The listing builds one solid part. Answer for the finished solid, in the listing's coordinates (mm). Face numbers are marked on the shaded views. Coordinates: 2 decimals unless noted, no trailing zeros. Order: outer loops, then holes, each group sorted by start corner. A loop starts at its lowest first (then second) coordinate and runs counter-clockwise, first axis right, second up. Notation, with made-up numbers: (65.5, 28.5) -> (115.5, 28.5) arc R17 ccw to (115.5, 48.5) -> close; hole circle Ø9 at (46, 37.25). An arc over 180 degrees is marked (long way). One line per question, with ' | ' between items.
from build123d import *

# Parameters (mm, degrees)
SKETCH1_W                = 39
SKETCH1_H                = 7.38
BOSS_EXTRUDE1_DEPTH      = 7.76
SKETCH2_R                = 2.4
CUT_EXTRUDE1_DEPTH       = 7.76
CUT_EXTRUDE2_OUTLINE_R   = 3.1
CUT_EXTRUDE2_OUTLINE_R_2 = 2.4
CUT_EXTRUDE2_DEPTH       = 0.8
CUT_EXTRUDE3_START       = 6.96
CUT_EXTRUDE3_OUTLINE_R   = 3.1
CUT_EXTRUDE3_OUTLINE_R_2 = 2.4
CUT_EXTRUDE3_DEPTH       = 0.8
LPATTERN3_COUNT          = 3
LPATTERN3_PITCH          = 7.79
LPATTERN6_COUNT          = 3
LPATTERN6_PITCH          = 7.79
FILLET1_R                = 3.69
FILLET2_R                = 3.69
FILLET3_R                = 3.69
FILLET4_R                = 3.69


# Read off the part's stored shape, not the designer's step: Cut-Extrude2, Cut-Extrude3
with BuildPart() as part:
    # Sketch1 → Boss-Extrude1 (new body)
    with BuildSketch(Plane.XY):
        with Locations((19.5, 3.69)):
            Rectangle(SKETCH1_W, SKETCH1_H)
    extrude(amount=BOSS_EXTRUDE1_DEPTH)

    # Sketch2 → Cut-Extrude1 (cut)
    with BuildSketch(Plane.XY.offset(7.76)):
        with Locations((19.5, 3.69)):
            Circle(SKETCH2_R)
    cut_extrude1 = extrude(amount=-CUT_EXTRUDE1_DEPTH, mode=Mode.SUBTRACT)

    # Cut-Extrude2 outline → Cut-Extrude2 (cut)
    with BuildSketch(Plane.XY):
        with Locations((19.5, 3.69)):
            Circle(CUT_EXTRUDE2_OUTLINE_R)
        with Locations((19.5, 3.69)):
            Circle(CUT_EXTRUDE2_OUTLINE_R_2, mode=Mode.SUBTRACT)
    cut_extrude2 = extrude(amount=CUT_EXTRUDE2_DEPTH, mode=Mode.SUBTRACT)

    # Cut-Extrude3 outline → Cut-Extrude3 (cut)
    with BuildSketch(Plane.XY.offset(CUT_EXTRUDE3_START)):
        with Locations((19.5, 3.69)):
            Circle(CUT_EXTRUDE3_OUTLINE_R)
        with Locations((19.5, 3.69)):
            Circle(CUT_EXTRUDE3_OUTLINE_R_2, mode=Mode.SUBTRACT)
    cut_extrude3 = extrude(amount=CUT_EXTRUDE3_DEPTH, mode=Mode.SUBTRACT)

    # LPattern3: Cut-Extrude1, Cut-Extrude2, Cut-Extrude3 ×3
    with Locations(*[(-i * LPATTERN3_PITCH, 0, 0) for i in range(1, LPATTERN3_COUNT)]):
        add(cut_extrude1, mode=Mode.SUBTRACT)
        add(cut_extrude2, mode=Mode.SUBTRACT)
        add(cut_extrude3, mode=Mode.SUBTRACT)

    # LPattern6: Cut-Extrude1, Cut-Extrude2, Cut-Extrude3 ×3
    with Locations(*[(i * LPATTERN6_PITCH, 0, 0) for i in range(1, LPATTERN6_COUNT)]):
        add(cut_extrude1, mode=Mode.SUBTRACT)
        add(cut_extrude2, mode=Mode.SUBTRACT)
        add(cut_extrude3, mode=Mode.SUBTRACT)

    # Fillet1
    fillet1_edges = [part.edges().sort_by_distance(p)[0] for p in [
        (0, 7.38, 3.88),
    ]]
    fillet(fillet1_edges, radius=FILLET1_R)

    # Fillet2
    fillet2_edges = [part.edges().sort_by_distance(p)[0] for p in [
        (0, 0, 3.88),
    ]]
    fillet(fillet2_edges, radius=FILLET2_R - 0.0001)  # a hair under: the kernel refuses the full size

    # Fillet3
    fillet3_edges = [part.edges().sort_by_distance(p)[0] for p in [
        (39, 7.38, 3.88),
    ]]
    fillet(fillet3_edges, radius=FILLET3_R)

    # Fillet4
    fillet4_edges = [part.edges().sort_by_distance(p)[0] for p in [
        (39, 0, 3.88),
    ]]
    fillet(fillet4_edges, radius=FILLET4_R - 0.0001)  # a hair under: the kernel refuses the full size


solid = part.part
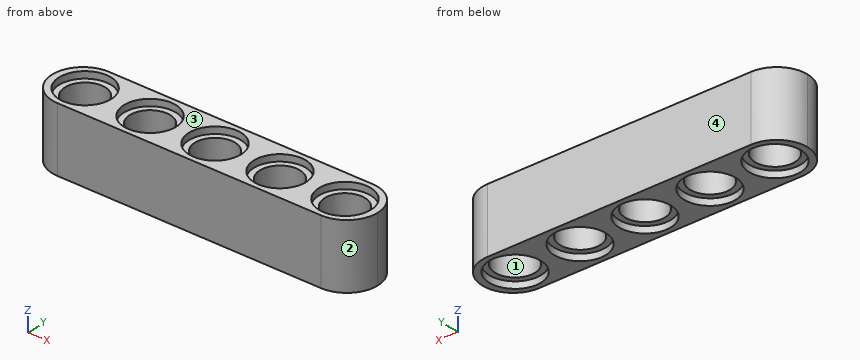
Item 1: Section D-D, the plane x = 5.5 is taken. Give the vertices of the cut face in (y, z), plus the area to 3 significant figures.
Computed values:
outline: (0, 0) -> (1.02, 0) -> (1.02, 0.8) -> (1.88, 0.8) -> (1.88, 6.96) -> (1.02, 6.96) -> (1.02, 7.76) -> (0, 7.76) -> close; (5.5, 0.8) -> (6.36, 0.8) -> (6.36, 0) -> (7.38, 0) -> (7.38, 7.76) -> (6.36, 7.76) -> (6.36, 6.96) -> (5.5, 6.96) -> close | area: 26.5 mm^2
Item 2: Determine the mould class of the marked faces 1, 2, 3 and 4 for opening direction Y: pulls with the +Y half, pulls with the -Y half, needs draft (parallel to the pull), parting line crosses it, or undercut.
Computed values:
face 1: undercut | face 2: pulls with the -Y half | face 3: needs draft | face 4: pulls with the +Y half
Item 3: Find the intervals of material crossed by L1, parallel to X at y = 3, z = 2; L2, parallel to Y at x = 11.71, z = 7.2; L3, parallel to X at y = 3.25, z = 2.5, in increasing order.
Computed values:
L1: x = 0.07 to 1.62, 6.22 to 9.41, 14.01 to 17.2, 21.8 to 24.99, 29.59 to 32.78, 37.38 to 38.93 | L2: y = 0 to 0.59, 6.79 to 7.38 | L3: x = 0.03 to 1.56, 6.28 to 9.35, 14.07 to 17.14, 21.86 to 24.93, 29.65 to 32.72, 37.44 to 38.97
Item 4: Section A-A, the plane x = 11.71 is taken. Give the vertices of the cut face in (y, z).
Computed values:
outline: (0, 0) -> (0.59, 0) -> (0.59, 0.8) -> (1.29, 0.8) -> (1.29, 6.96) -> (0.59, 6.96) -> (0.59, 7.76) -> (0, 7.76) -> close; (6.09, 0.8) -> (6.79, 0.8) -> (6.79, 0) -> (7.38, 0) -> (7.38, 7.76) -> (6.79, 7.76) -> (6.79, 6.96) -> (6.09, 6.96) -> close
Item 5: Section B-B, the plane z = 3.75 is taken. Count the separate pieces of the cut face and the enclosed holes in it, plus the area to 3 significant figures.
Computed values:
separate pieces: 1 | enclosed holes: 5 | area: 186 mm^2
Item 6: This flat-tipped pin is pushed along its axis until it touches: pin 1 Ø3 at (y, z) = (4, 6.5) entering from -X. Where does it stop, or does it pass through?
Computed values:
pin 1: stops at x = 0
